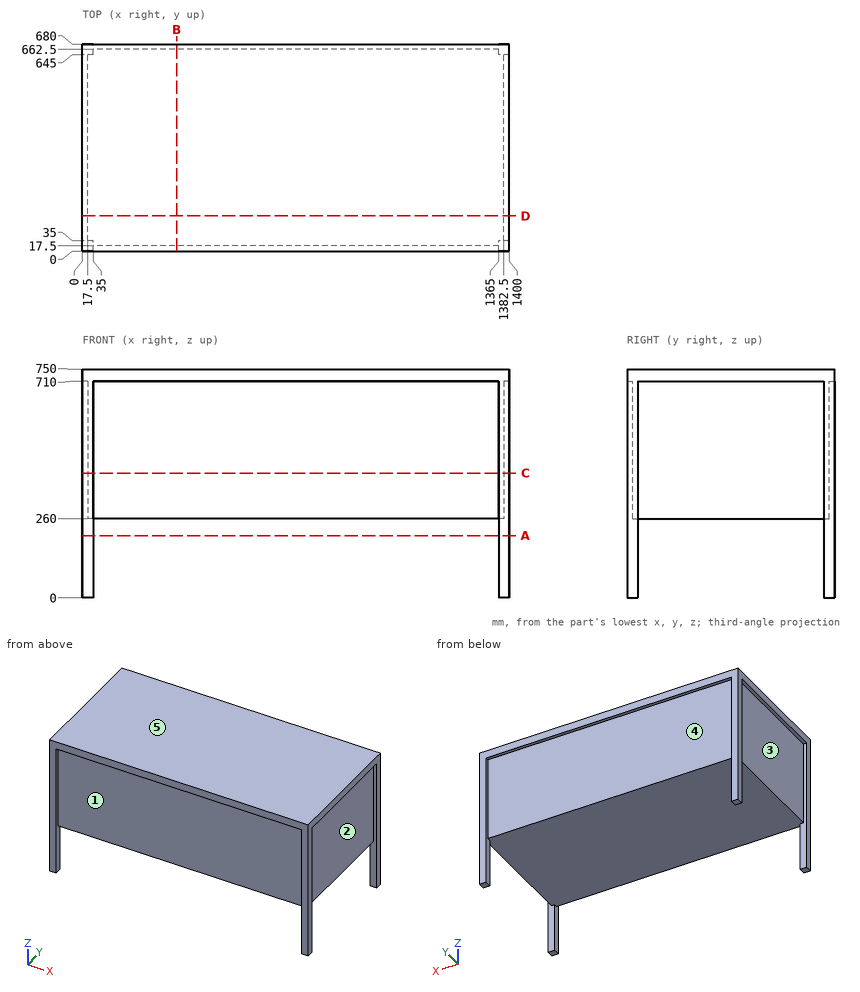
For this review, use the dimensioned drawing (mm, ordinates from the lowest corner) and the shaded views. A direction names the side the tool comes from. Give positions to 0.01 mm unless a question says otherwise; leave off trailing zeros. Write each loop counter-clockwise with the first axis right and the second up, starting at its lowest first coordinate (ties: lowest second). Pieces come first, ordered by that corner, then holes. Notation, with made-up numbers: M 13,32.5 L 59,32.5 A22 cw 59,45.5 Z; hole C 19,61 d10. An arc over 180 degrees is marked long. Answer as a JSON object with one key per item and string values. Group by question number.
1) Mouldability with a two-part tool opening along X and no side actions: class the marked faces 3, 4 and 5 as released by +X, released by -X, zero draft, split by the parting line, or undercut.
2) We need section A-A (z = 204.5). Give the boundary of the cut face in (x, y).
3) Tool access review of the marked faces 1 and 2: name each direction out of +Z, -Z, +X, -X, +Y, -Y from which nothing blocks a thin tool from reaching the whole face with its end or side.
4) We need section C-C (z = 409). Give the boundary of the cut face in (x, y), and give its area (3 significant figures).
5) Clearance check with flat-ended pins moving along their axes: pin 1 Ø9 at (x, y) = (7.5, 329) entering from -Z; pin 2 Ø6 at (y, z) = (489.5, 591.5) entering from +X; pin 3 Ø12 at (x, z) = (559.5, 375) entering from -Y. State where each tip first meets the part, or that it passes through.
6) We need section D-D (y = 116). Give the boundary of the cut face in (x, z), and give its area (3 significant figures).
7) For line 1 along Y through (x, z) = (100, 573.5); line 2 along Z through (x, y) = (552, 112); line 3 along X through (y, z) = (137.5, 323), list the stretches that pass through material, from the lowest coordinate up.
8) We need section B-B (x = 308.5). Give the boundary of the cut face in (y, z), and give its area (3 significant figures).
Answer key:
{
 "1": {"face 3": "released by -X", "face 4": "undercut", "face 5": "zero draft"},
 "2": {"outline": "M 0,0 L 35,0 L 35,35 L 0,35 Z; M 0,645 L 35,645 L 35,680 L 0,680 Z; M 1365,0 L 1400,0 L 1400,35 L 1365,35 Z; M 1365,645 L 1400,645 L 1400,680 L 1365,680 Z"},
 "3": {"face 1": "-Z, -Y", "face 2": "-Z, +X"},
 "4": {"outline": "M 0,0 L 35,0 L 35,17.5 L 1365,17.5 L 1365,0 L 1400,0 L 1400,35 L 1382.5,35 L 1382.5,645 L 1400,645 L 1400,680 L 1365,680 L 1365,662.5 L 35,662.5 L 35,680 L 0,680 L 0,645 L 17.5,645 L 17.5,35 L 0,35 Z", "area": "884,000 mm²"},
 "5": {"pin 1": "stops at z = 710", "pin 2": "stops at x = 1382.5", "pin 3": "stops at y = 17.5"},
 "6": {"outline": "M 0,710 L 17.5,710 L 17.5,260 L 1382.5,260 L 1382.5,710 L 1400,710 L 1400,750 L 0,750 Z", "area": "670,000 mm²"},
 "7": {"line 1": "y = 17.5 to 662.5", "line 2": "z = 260 to 750", "line 3": "x = 17.5 to 1382.5"},
 "8": {"outline": "M 0,710 L 17.5,710 L 17.5,260 L 662.5,260 L 662.5,710 L 680,710 L 680,750 L 0,750 Z", "area": "317,000 mm²"}
}
